Autodesk Inventor part; units mm, degrees
ref_plane "YZ Plane" through (0, 0, 0) normal (1, 0, 0) x (0, 1, 0)
ref_plane "XZ Plane" through (0, 0, 0) normal (0, 1, 0) x (-1, 0, 0)
ref_plane "XY Plane" through (0, 0, 0) normal (0, 0, 1) x (1, 0, 0)
sketch "Sketch1" plane through (0, 0, 0) normal (1, 0, 0) x (0, 1, 0)
  line L0 (0, 0) -> (22.225, 0)
  line L1 (22.225, 0) -> (22.225, -59.69)
  line L2 (0, -59.69) -> (0, 0)
  line L3 (4.7625, -59.69) -> (5.9323, -59.69)
  line L4 (4.7625, -59.69) -> (4.7625, -4.7625)
  line L5 (4.7625, -4.7625) -> (17.4625, -4.7625)
  line L6 (17.4625, -4.7625) -> (17.4625, -59.69)
  line L7 (22.225, -59.69) -> (17.4625, -59.69)
  line L8 (4.7625, -59.69) -> (0, -59.69)
  dimension "d1" = 59.69
  dimension "d4" = 12.7
  dimension "d6" = 4.7625
  dimension "d15" = 59.69
  dimension "d22" = 4.7625
  dimension "d24" = 4.7625
extrude "Extrusion1" add sketch "Sketch1" along normal blind 12.7
sketch "Sketch2" plane through (0, 22.225, 0) normal (0, 1, 0) x (1, 0, 0)
  circle A0 centre (6.35, 53.34) radius 2.4765
  line L0 (0, 0) -> (0, 59.69)
  line L1 (0, 0) -> (12.7, 0)
  line L2 (12.7, 59.69) -> (12.7, 0)
  line L3 (0, 59.69) -> (12.7, 59.69)
  point P0 (0, 0)
  dimension "d9" = 4.953
  dimension "d10" = 12.7
  dimension "d11" = 6.35
  dimension "d16" = 6.35
extrude "Extrusion2" cut sketch "Sketch2" against normal blind 25.4 contours A0
sketch "Sketch3" plane through (0, 4.7625, -4.7625) normal (0, 0, -1) x (-1, 0, 0)
  line L0 (0, 12.7) -> (0, 0)
  line L1 (0, 12.7) -> (-12.7, 12.7)
  line L2 (-12.7, 0) -> (-12.7, 12.7)
  line L3 (0, 0) -> (-12.7, 0)
  line L4 (0, 0) -> (-12.7, 0)
  line L5 (0, 0) -> (0, -4.7625)
  line L6 (0, 0) -> (-12.7, 0)
  line L7 (-12.7, -4.7625) -> (-12.7, 0)
  line L8 (0, -4.7625) -> (-12.7, -4.7625)
  circle A0 centre (-6.35, 6.35) radius 4.7625
  point P0 (0, -4.7625)
  dimension "d17" = 9.525
  dimension "d18" = 6.35
  dimension "d19" = 6.35
  dimension "d23" = 12.7
extrude "Extrusion3" cut sketch "Sketch3" against normal blind 3.175 contours A0
sketch "Sketch4" plane through (0, 0, 0) normal (0, 0, 1) x (1, 0, 0)
  line L0 (0, 0) -> (0, 22.225)
  line L1 (0, 0) -> (12.7, 0)
  line L2 (12.7, 22.225) -> (12.7, 0)
  line L3 (0, 22.225) -> (12.7, 22.225)
  circle A0 centre (6.35, 11.1125) radius 1.778
  dimension "d25" = 3.556
extrude "Extrusion4" cut sketch "Sketch4" against normal blind 25.4 contours A0
fillet "Fillet2" radius 0.381 22 edges at (12.7, 22.225, -29.845) (12.7, 17.4625, -32.2263) (0, 22.225, -29.845) (12.7, 11.1125, 0) (12.7, 11.1125, -4.7625) (12.7, 4.7625, -32.2263) (12.7, 0, -29.845) (12.7, 19.8438, -59.69) (12.7, 2.3813, -59.69) (6.35, 22.225, 0) (0, 11.1125, 0) (6.35, 0, 0) (6.35, 22.225, -59.69) (6.35, 4.7625, -59.69) (0, 17.4625, -32.2263) (0, 11.1125, -4.7625) (0, 4.7625, -32.2263) (6.35, 17.4625, -59.69) (0, 19.8438, -59.69) (0, 2.3813, -59.69) (0, 0, -29.845) (6.35, 0, -59.69)
equation "\"d15\" = d1"
equation "\"d11\" = 0.5 * d10"
equation "\"d16\" = d11"
equation "\"d18\" = 0.5 * d23"
properties part number "TensionerAxleHolder"
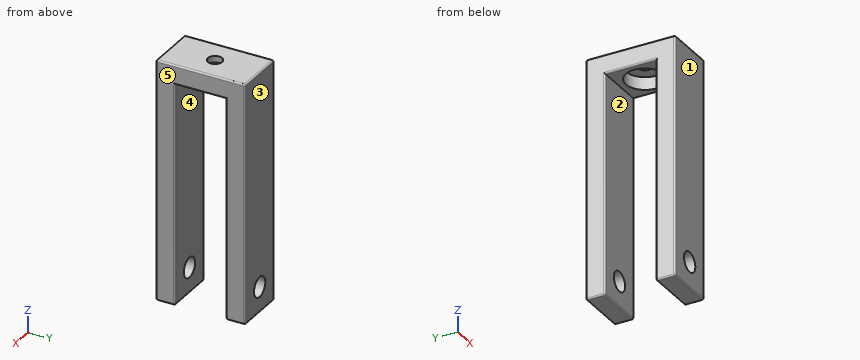
The model under review builds one solid part; all positions refer to its coordinate system, in mm. Face numbers are marked on the shaded views. A direction names the side the tool comes from. Round coordinates to 2 decimals unless told otherwise and drop trailing zeros. Write each loop counter-clockwise with the first axis right and the second up, starting at its lowest first coordinate (ties: lowest second). Pieces come first, ordered by that corner, then holes.
(1) We need section A-A on z = -19.5. Give the boundary of the cut face in (x, y) (1 decimal), and give its area (3 significant figures).
(2) We need section B-B on x = 6.35. Give the number of separate pieces and of enclosed holes in the cut face, and give its area (3 significant figures).
(3) Mouldability with a two-part tool opening along Y and no side actions: class the marked faces 3, 4 and 5 as +Y half, -Y half, draft (parallel to the pull), parting line (faces both ways), or undercut.
(4) We need section C-C on z = -53.34. Give the boundary of the cut face in (x, y) (1 decimal), and give its area (3 significant figures).
(5) Wall thickness on L1, parallel to Y at x = 7.5, z = -51 (1 decimal); L2, parallel to Z at x = 6.35, y = 3.1; L3, parallel to Y at x = 6.35, z = -3.3 (3 decimals): over which ranges is each line inside the solid? List them lowest first.
(6) Insertion check: pin 1 (6 mm diameter, centred on x = 7.5, y = 9, fed in from -Z); pin 2 (4 mm diameter, centred on x = 6.35, z = -53.34, fed in from +Y). Each pin has a flat end and moves straight along its axis. Give the tip position at first contact, or say it passes through.
(7) Machinability: for the marked faces 1 and 2, which of the approach directions +Z, -Z, +X, -X, +Y, -Y give a long, thin tool a straight path to every point of the face, cutting with its end or side? Answer none if there is none.
(8) We need section D-D on y = 7.75. Give the boundary of the cut face in (x, z), and give its area (3 significant figures).
Findings below:
1. outline: (0, 0.4) arc R0.4 ccw to (0.4, 0) - (12.3, 0) arc R0.4 ccw to (12.7, 0.4) - (12.7, 4.4) arc R0.4 ccw to (12.3, 4.8) - (0.4, 4.8) arc R0.4 ccw to (0, 4.4) - close; (0, 17.8) arc R0.4 ccw to (0.4, 17.5) - (12.3, 17.5) arc R0.4 ccw to (12.7, 17.8) - (12.7, 21.8) arc R0.4 ccw to (12.3, 22.2) - (0.4, 22.2) arc R0.4 ccw to (0, 21.8) - close
1. area: 121 mm2
2. separate pieces: 4
2. enclosed holes: 0
2. area: 546 mm2
3. face 3: +Y half
3. face 4: undercut
3. face 5: draft
4. outline: (0, 0.4) arc R0.4 ccw to (0.4, 0) - (3.9, 0) - (3.9, 4.8) - (0.4, 4.8) arc R0.4 ccw to (0, 4.4) - close; (0, 17.8) arc R0.4 ccw to (0.4, 17.5) - (3.9, 17.5) - (3.9, 22.2) - (0.4, 22.2) arc R0.4 ccw to (0, 21.8) - close; (8.8, 0) - (12.3, 0) arc R0.4 ccw to (12.7, 0.4) - (12.7, 4.4) arc R0.4 ccw to (12.3, 4.8) - (8.8, 4.8) - close; (8.8, 17.5) - (12.3, 17.5) arc R0.4 ccw to (12.7, 17.8) - (12.7, 21.8) arc R0.4 ccw to (12.3, 22.2) - (8.8, 22.2) - close
4. area: 73.5 mm2
5. L1: y = 0 to 4.8, 17.5 to 22.2
5. L2: z = -59.69 to -55.82, -50.86 to 0
5. L3: y = 0 to 6.35, 15.875 to 22.225
6. pin 1: stops at z = -4.76
6. pin 2: passes through
7. face 1: +Z, -Z, +X, -X, -Y
7. face 2: -Z, +X, -X
8. outline: (0, -4.38) arc R0.38 ccw to (0.38, -4.76) - (2.98, -4.76) - (2.98, -1.59) - (9.72, -1.59) - (9.72, -4.76) - (12.32, -4.76) arc R0.38 ccw to (12.7, -4.38) - (12.7, -0.38) arc R0.38 ccw to (12.32, 0) - (0.38, 0) arc R0.38 ccw to (0, -0.38) - close
8. area: 38.9 mm2
